Check sheet for the drawn part. Datum: minimum x, y, z corner. Units: mm. Give positions to 0.01 mm unless a question says otherwise; leave off trailing zeros. Order: outer loops, then holes, each group sorted by start corner. A loop starts at its lowest first (then second) coordinate and runs counter-clockwise, first axis right, second up. Notation, with made-up numbers: (24, 38.25) -> (43, 38.25) arc R14 cw to (43, 54.25) -> close; hole circle Ø10 at (60.5, 16). An arc over 180 degrees is marked (long way). One line per question, with ' | ' between items. Start each with the question number.
Q1. Material ranges on probe 1 along Y at (x, z) = (26, 2.5); probe 2 along X at (y, z) = (27.5, 2); probe 3 along Y at (x, z) = (25, 6), recorded low to high. Write a range as [from, to].
Q2. Mould release check, pull along X, two halves, no side actions. Record for the marked faces 1, 2 and 3: released by +X, released by -X, zero draft, split by the parting line, or undercut.
Q3. Section check A-A on x = 64. Record the cut outline in (y, z), plus the area to 3 significant figures.
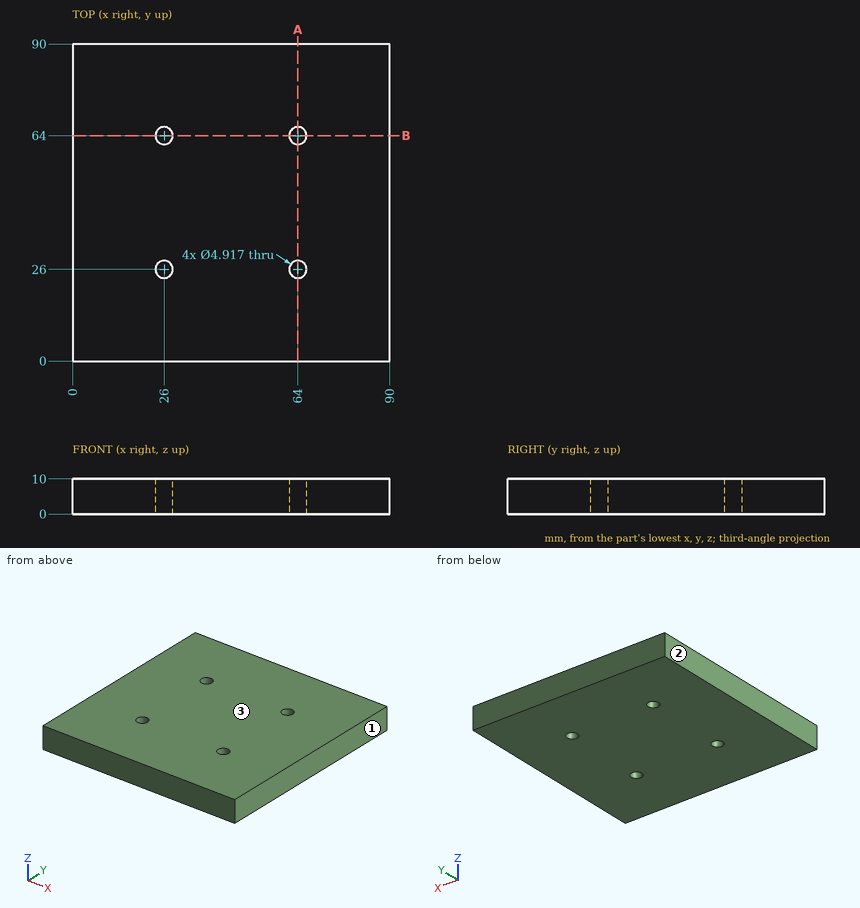
Filled in:
1) probe 1: [0, 23.54], [28.46, 61.54], [66.46, 90] | probe 2: [0, 24.05], [27.95, 62.05], [65.95, 90] | probe 3: [0, 23.75], [28.25, 61.75], [66.25, 90]
2) face 1: released by +X | face 2: released by -X | face 3: zero draft
3) outline: (0, 0) -> (23.54, 0) -> (23.54, 10) -> (0, 10) -> close; (28.46, 0) -> (61.54, 0) -> (61.54, 10) -> (28.46, 10) -> close; (66.46, 0) -> (90, 0) -> (90, 10) -> (66.46, 10) -> close | area: 802 mm²
